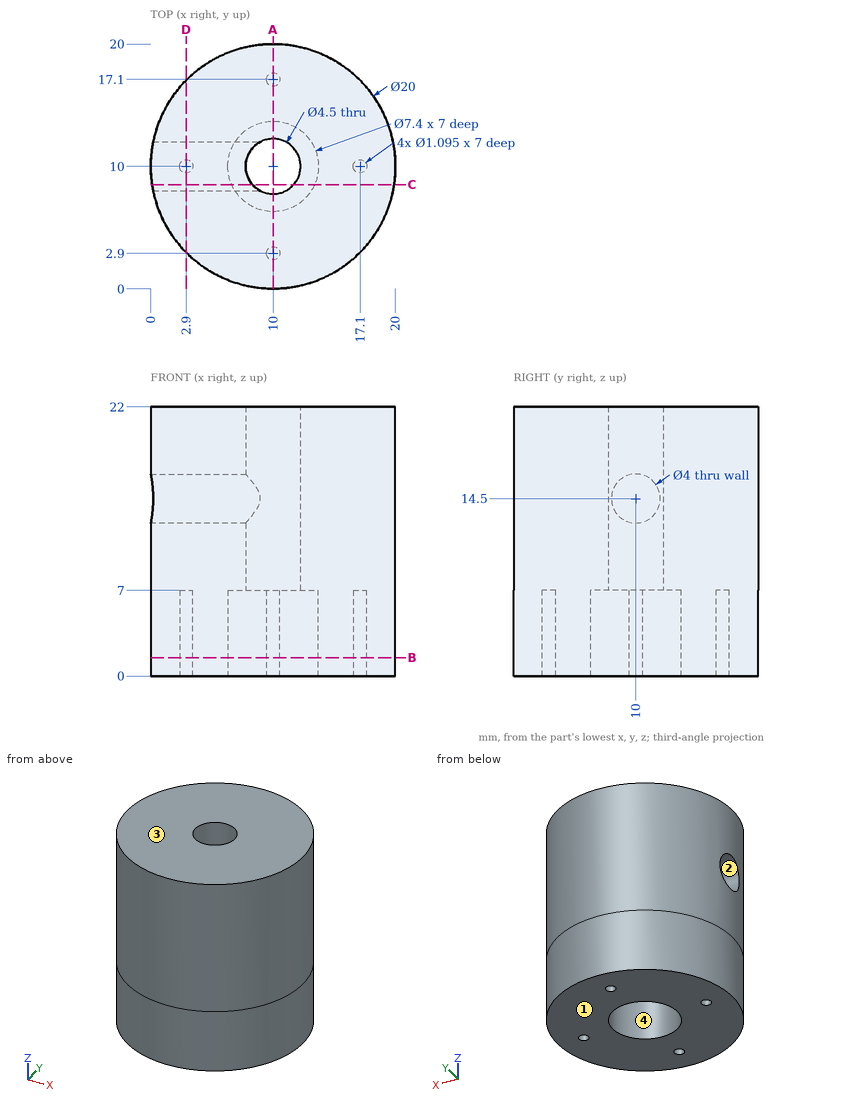
Check sheet for the drawn part. Datum: minimum x, y, z corner. Units: mm. A direction names the side the tool comes from. Round coordinates to 2 decimals unless told otherwise and drop trailing zeros. Order: outer loops, then holes, each group sorted by start corner. A loop starts at its lowest first (then second) coordinate and runs counter-clockwise, first axis right, second up.
1) Section check A-A (x = 10). Record the boundary of the cut face in (y, z), and give its area (3 significant figures).
2) Go/stop test with flat-tipped pins: pin 1 Ø1 at (x, y) = (10, 2.9) entering from -Z; pin 2 Ø5 at (y, z) = (10, 14.5) entering from -X; pin 3 Ø1 at (y, z) = (8.5, 14.5) entering from +X; pin 4 Ø8 at (y, z) = (14.5, 16.5) entering from +X. Record where each tip stops, or that it passes through.
3) Scan lines: line 1 (Z direction, x = 12, y = 12); line 2 (Y direction, x = 10, z = 19.25); line 3 (X direction, y = 10.25, z = 1.5) (1 decimal). Record each from-to range of solid material in increasing order.
4) Section check C-C (y = 8.5). Record the boundary of the cut face in (x, z), and give its area (3 significant figures).
5) Tool access check on the marked faces 1 and 2. Record the directions out of +Z, -Z, +X, -X, +Y, -Y that give a thin tool (end or side, any length) a straight path to the whole face; none if there is none.
6) Section check B-B (z = 1.5). Record the boundary of the cut face in (x, y) (1 decimal).
7) Section check D-D (x = 2.9). Record the boundary of the cut face in (y, z), and give its area (3 significant figures).
8) Mould release check, pull along X, two halves, no side actions. Record for the marked faces 3 and 4: +X half, -X half, draft (parallel to the pull), parting line (faces both ways), or undercut.
Result:
1. outline: (0, 0) - (2.35, 0) - (2.35, 7) - (3.45, 7) - (3.45, 0) - (6.3, 0) - (6.3, 7) - (7.75, 7) - (7.75, 22) - (0, 22) - close; (12.25, 7) - (13.7, 7) - (13.7, 0) - (16.55, 0) - (16.55, 7) - (17.65, 7) - (17.65, 0) - (20, 0) - (20, 22) - (12.25, 22) - close
1. area: 305 mm2
2. pin 1: stops at z = 7
2. pin 2: stops at x = 0
2. pin 3: stops at x = 19.95
2. pin 4: stops at x = 19.99
3. line 1: z = 7 to 22
3. line 2: y = 0 to 7.75, 12.25 to 20
3. line 3: x = 0 to 2.4, 3.4 to 6.3, 13.7 to 16.6, 17.6 to 20
4. outline: (0.11, 0) - (6.62, 0) - (6.62, 7) - (8.32, 7) - (8.32, 13.18) - (0.11, 13.18) - close; (0.11, 15.82) - (8.32, 15.82) - (8.32, 22) - (0.11, 22) - close; (11.68, 7) - (13.38, 7) - (13.38, 0) - (19.89, 0) - (19.89, 22) - (11.68, 22) - close
4. area: 316 mm2
5. face 1: -Z, +X, -X, +Y, -Y
5. face 2: -X
6. outline: circle Ø20 at (10, 10); hole circle Ø1.1 at (2.9, 10); hole circle Ø7.4 at (10, 10); hole circle Ø1.1 at (10, 2.9); hole circle Ø1.1 at (10, 17.1); hole circle Ø1.1 at (17.1, 10)
7. outline: (2.96, 0) - (9.45, 0) - (9.45, 7) - (10.55, 7) - (10.55, 0) - (17.04, 0) - (17.04, 22) - (2.96, 22) - close; hole circle Ø4 at (10, 14.5)
7. area: 290 mm2
8. face 3: draft
8. face 4: undercut
